```python
from build123d import *

# Parameters (mm, degrees)
SKETCH1_W           = 255.45
SKETCH1_H           = 260.35
BOSS_EXTRUDE1_DEPTH = 3.175
SKETCH2_W           = 255.45
SKETCH2_H           = 6.35
BOSS_EXTRUDE2_DEPTH = 12.7
CUT_EXTRUDE1_DEPTH  = 16.875
SKETCH5_W           = 54.590141408
SKETCH5_H           = 33.859166417
CUT_EXTRUDE2_DEPTH  = 256.45
SKETCH8_R           = 1.55
SKETCH8_R_2         = 1.6999966
SKETCH8_R_3         = 1.5499969
SKETCH8_R_4         = 1.05
CUT_EXTRUDE7_DEPTH  = 4.175
SKETCH9_W           = 50.8
SKETCH9_H           = 76.2
CUT_EXTRUDE8_DEPTH  = 4.175
FILLET1_R           = 12.7
CUT_EXTRUDE9_DEPTH  = 4.175


with BuildPart() as part:
    # Sketch1 → Boss-Extrude1 (new body)
    with BuildSketch(Plane(origin=(0, 0, 0), x_dir=(0, 0, -1), z_dir=(1, 0, 0))):
        Rectangle(SKETCH1_W, SKETCH1_H)
    extrude(amount=BOSS_EXTRUDE1_DEPTH)

    # Sketch2 → Boss-Extrude2 (add)
    with BuildSketch(Plane(origin=(3.175, 0, 0), x_dir=(0, 0, -1), z_dir=(1, 0, 0))):
        with Locations((0, 127)):
            Rectangle(SKETCH2_W, SKETCH2_H)
    extrude(amount=BOSS_EXTRUDE2_DEPTH)

    # Sketch3 → Cut-Extrude1 (cut, through all)
    with BuildSketch(Plane.ZY):
        with BuildLine():
            Line((-105.025, -73.025), (-37.375, -73.025))
            ThreePointArc((-37.375, -73.025), (-24.675, -85.725), (-37.375, -98.425))
            Line((-37.375, -98.425), (-105.025, -98.425))
            ThreePointArc((-105.025, -98.425), (-117.725, -85.725), (-105.025, -73.025))
        make_face()
    extrude(amount=-CUT_EXTRUDE1_DEPTH, mode=Mode.SUBTRACT)

    # Sketch5 → Cut-Extrude2 (cut, through all)
    with BuildSketch(Plane(origin=(0, 0, -127.725), x_dir=(-1, 0, 0), z_dir=(0, 0, -1))):
        with Locations((-30.470070704, 140.754583209)):
            Rectangle(SKETCH5_W, SKETCH5_H)
    extrude(amount=-CUT_EXTRUDE2_DEPTH, mode=Mode.SUBTRACT)

    # Sketch8 → Cut-Extrude7 (cut, through all)
    with BuildSketch(Plane.ZY):
        with Locations((115.025, 9.525)):
            Circle(SKETCH8_R)
        with Locations((-53.205, 11.825)):
            Circle(SKETCH8_R_2)
        with Locations((-42.9049952, -10.375)):
            Circle(SKETCH8_R_3)
        with Locations((-44.605, 18.925)):
            Circle(SKETCH8_R_4)
        with Locations((-44.605, 12.425)):
            Circle(SKETCH8_R_4)
    extrude(amount=-CUT_EXTRUDE7_DEPTH, mode=Mode.SUBTRACT)

    # Sketch9 → Cut-Extrude8 (cut, through all)
    with BuildSketch(Plane.ZY):
        with Locations((102.325, -92.075)):
            Rectangle(SKETCH9_W, SKETCH9_H)
    extrude(amount=-CUT_EXTRUDE8_DEPTH, mode=Mode.SUBTRACT)

    # Fillet1
    fillet1_edges = [part.edges().sort_by_distance(p)[0] for p in [
        (1.5875, -53.975, 76.925),
    ]]
    fillet(fillet1_edges, radius=FILLET1_R)

    # Sketch10 → Cut-Extrude9 (cut, through all)
    with BuildSketch(Plane.ZY):
        with BuildLine():
            ThreePointArc((-15.792035743, -58.127079483), (-9.357313119, -60.175), (-7.309392602, -53.740277376))
            ThreePointArc((-7.309392602, -53.740277376), (-17.536268555, -27.834189149), (-22.341982218, -0.400277376))
            ThreePointArc((-22.341982218, -0.400277376), (-27.448590626, 4.018114216), (-31.866982218, -1.088494191))
            ThreePointArc((-31.866982218, -1.088494191), (-26.728041298, -30.424668105), (-15.792035743, -58.127079483))
        make_face()
    extrude(amount=-CUT_EXTRUDE9_DEPTH, mode=Mode.SUBTRACT)


solid = part.part
```
Could you check a few things on this model? Use its own coordinates, in mm. A direction names the side the tool comes from. Coordinates: 2 decimals unless noted, no trailing zeros. Loops run counter-clockwise (first coordinate to the right, second up) from the corner with the lowest first, then second, coordinate; pieces in that order, holes last.
1) Imagine slicing it at C-C (y = -23). List the corners of the cut face in (x, z) for me (3 decimals), and give its area (3 significant figures).
Reported:
outline: (0, -127.725) - (3.175, -127.725) - (3.175, -28.614) - (0, -28.614) - close; (0, -18.804) - (3.175, -18.804) - (3.175, 127.725) - (0, 127.725) - close
area: 780 mm2
2) Thinking about a two-plate mould opening in Z: for faces 3 (the face through (1.57, -30.02, -26.84)), 4 (the face through (1.61, -57.6, 80.74)), 5 (the face through (3.175, 2, 2)), which applies, released by +Z, released by -Z, zero draft, split by the parting line, or undercut?
Reported:
face 3: undercut
face 4: released by +Z
face 5: zero draft
3) Imagine slicing it at B-B (z = -111.5). List the corners of the cut face in (x, y) for me (3 decimals), and give its area (3 significant figures).
Reported:
outline: (0, -130.175) - (3.175, -130.175) - (3.175, -96.65) - (0, -96.65) - close; (0, -74.8) - (3.175, -74.8) - (3.175, 130.175) - (0, 130.175) - close
area: 757 mm2
4) Which directions (+Z, -Z, +X, -X, +Y, -Y) give clear straight access to the entire face, cutting with the end or side of a thin tool? Please do faces 1 (the face through (1.57, -28.21, -17.43)), 2 (the face through (0, 2, 2)).
Reported:
face 1: +X, -X
face 2: +Z, -Z, -X, +Y, -Y
5) Imagine slicing it at D-D (x = 1.7). State how many separate pieces and enclosed holes the cut face has, and give its area (3 significant figures).
Reported:
separate pieces: 1
enclosed holes: 7
area: 59,800 mm2
6) Please list where these lines run through material, in increasing order: line 1 along Y through (x, z) = (1.75, -99.5) (3 decimals); line 2 along Z through (x, y) = (0.6, -41) (3 decimals); line 3 along Y through (x, z) = (1.5, 92.5) (3 decimals).
Reported:
line 1: y = -130.175 to -98.425, -73.025 to 130.175
line 2: z = -127.725 to -23.312, -13.098 to 127.725
line 3: y = -53.975 to 130.175
7) Imagine slicing it at A-A (z = -28.5). List the corners of the cut face in (x, y) for me (3 decimals), and give its area (3 significant figures).
Reported:
outline: (0, -130.175) - (3.175, -130.175) - (3.175, -94.809) - (0, -94.809) - close; (0, -76.641) - (3.175, -76.641) - (3.175, -23.497) - (0, -23.497) - close; (0, 3.822) - (3.175, 3.822) - (3.175, 130.175) - (0, 130.175) - close
area: 682 mm2
8) Will these pins go through, and if not, where does the flat tip stop? pin 1 Ø4 at (y, z) = (9.525, 115.025) entering from -X; pin 2 Ø1.7 at (y, z) = (18.925, -44.605) entering from -X; pin 3 Ø1 at (x, y) = (2, -105) entering from +Z (3 decimals).
Reported:
pin 1: stops at x = 0
pin 2: passes through
pin 3: stops at z = 76.925
